The listing builds one solid part. Answer for the finished solid, in the listing's coordinates (mm). Round coordinates to 2 decimals unless told otherwise and drop trailing zeros. Write each loop counter-clockwise with the first axis right and the second up, starting at its lowest first coordinate (ties: lowest second). Pieces come first, ordered by that corner, then holes. Notation, with made-up numbers: M 11.5,54.25 L 47.5,54.25 A17 cw 47.5,78.25 Z; hole C -21.75,-40 d3. An arc over 180 degrees is marked long. One line per item, written item: value. Start each with the question number.
(1) Consider probe 1 along Z at (x, y) = (138, 0.7); probe 2 along Z at (x, y) = (254, 1.85); probe 3 along Z at (x, y) = (268.5, 2). Determine where each line is inside the solid, lowest interval first.
(2) Given P1, Ø3, axis at x = 253.5, z = -110, coming from the +Y side; P2, Ø4.5, axis at x = 253.5, z = -45, coming from the +Y side; P3, Ø1.5, axis at y = 1.5, z = -4.5, coming from the +X side; P4, Ø1.5, axis at y = 2, z = -98, coming from the -X side, each flat-ended and moving along its own axis, determine where each tip first touches the part or whether it passes through.
(3) Section A-A (z = -74.5) is taken. Determine the outline of the cut face in (x, y), plus the area to 3 significant figures.
(4) Section D-D (x = 67) is taken. Determine the outline of the cut face in (y, z).
(5) Section B-B (x = 290) is taken. Determine the outline of the cut face in (y, z).
(6) Section C-C (y = 2.15) is taken. State how many separate pieces and enclosed holes the cut face has, plus the area to 3 significant figures.
```python
from build123d import *

# Parameters (mm, degrees)
ESQUISSE1_R      = 2.5
EXTRUSION1_DEPTH = 3
CONG_1_R         = 15
EXTRUSION2_REACH = 5
ESQUISSE2_W      = 300
ESQUISSE2_H      = 3
ESQUISSE2_W_2    = 3
ESQUISSE2_H_2    = 93
ESQUISSE3_R      = 2
EXTRUSION3_DEPTH = 3


with BuildPart() as part:
    # Esquisse1 → Extrusion1 (new body)
    with BuildSketch(Plane(origin=(0, 0, 0), x_dir=(1, 0, 0), z_dir=(0, 1, 0))):
        Polygon((0, 0), (24, 0), (24, 14), (306, 14), (306, 0), (330, 0), (330, 123), (0, 123), align=None)
        with Locations((10, 113)):
            Circle(ESQUISSE1_R, mode=Mode.SUBTRACT)
        with Locations((320, 113)):
            Circle(ESQUISSE1_R, mode=Mode.SUBTRACT)
        with Locations((10, 12)):
            Circle(ESQUISSE1_R, mode=Mode.SUBTRACT)
        with Locations((320, 12)):
            Circle(ESQUISSE1_R, mode=Mode.SUBTRACT)
        with BuildLine():
            Line((280, 93), (280, 54))
            ThreePointArc((280, 54), (290, 44), (300, 54))
            Line((300, 54), (300, 93))
            ThreePointArc((300, 93), (290, 103), (280, 93))
        make_face(mode=Mode.SUBTRACT)
        with BuildLine():
            Line((30, 93), (30, 54))
            ThreePointArc((30, 54), (40, 44), (50, 54))
            Line((50, 54), (50, 93))
            ThreePointArc((50, 93), (40, 103), (30, 93))
        make_face(mode=Mode.SUBTRACT)
    extrude(amount=EXTRUSION1_DEPTH)

    # Congé1
    cong_1_edges = [part.edges().sort_by_distance(p)[0] for p in [
        (0, 1.5, -123),
        (330, 1.5, -123),
        (330, 1.5, 0),
        (0, 1.5, 0),
    ]]
    fillet(cong_1_edges, radius=CONG_1_R)

    # Esquisse2 → Extrusion2 (cut, up to next)
    with BuildSketch(Plane(origin=(0, 3, 0), x_dir=(1, 0, 0), z_dir=(0, 1, 0)), mode=Mode.PRIVATE) as extrusion2_sk1:
        with Locations((165, 121.5)):
            Rectangle(ESQUISSE2_W, ESQUISSE2_H)
    extrusion2_tool1 = extrude(extrusion2_sk1.sketch, amount=-EXTRUSION2_REACH, mode=Mode.PRIVATE) & part.part
    add(extrusion2_tool1.solids().sort_by_distance((165, 3, -121.5))[0], mode=Mode.SUBTRACT)
    # Esquisse2 → Extrusion2 (cut, up to next)
    with BuildSketch(Plane(origin=(0, 3, 0), x_dir=(1, 0, 0), z_dir=(0, 1, 0)), mode=Mode.PRIVATE) as extrusion2_sk2:
        with Locations((1.5, 61.5)):
            Rectangle(ESQUISSE2_W_2, ESQUISSE2_H_2)
    extrusion2_tool2 = extrude(extrusion2_sk2.sketch, amount=-EXTRUSION2_REACH, mode=Mode.PRIVATE) & part.part
    add(extrusion2_tool2.solids().sort_by_distance((1.5, 3, -61.5))[0], mode=Mode.SUBTRACT)
    # Esquisse2 → Extrusion2 (cut, up to next)
    with BuildSketch(Plane(origin=(0, 3, 0), x_dir=(1, 0, 0), z_dir=(0, 1, 0)), mode=Mode.PRIVATE) as extrusion2_sk3:
        with Locations((328.5, 61.5)):
            Rectangle(ESQUISSE2_W_2, ESQUISSE2_H_2)
    extrusion2_tool3 = extrude(extrusion2_sk3.sketch, amount=-EXTRUSION2_REACH, mode=Mode.PRIVATE) & part.part
    add(extrusion2_tool3.solids().sort_by_distance((328.5, 3, -61.5))[0], mode=Mode.SUBTRACT)

    # Esquisse3 → Extrusion3 (cut)
    with BuildSketch(Plane(origin=(0, 3, 0), x_dir=(1, 0, 0), z_dir=(0, 1, 0))):
        with Locations((76.5, 110)):
            Circle(ESQUISSE3_R)
        with Locations((253.5, 110)):
            Circle(ESQUISSE3_R)
        with Locations((76.5, 24)):
            Circle(ESQUISSE3_R)
        with Locations((253.5, 24)):
            Circle(ESQUISSE3_R)
        with Locations((61.5, 110)):
            Circle(ESQUISSE3_R)
        with Locations((106.5, 110)):
            Circle(ESQUISSE3_R)
        with Locations((61.5, 87)):
            Circle(ESQUISSE3_R)
        with Locations((106.5, 87)):
            Circle(ESQUISSE3_R)
        with Locations((61.5, 47)):
            Circle(ESQUISSE3_R)
        with Locations((106.5, 47)):
            Circle(ESQUISSE3_R)
        with Locations((106.5, 24)):
            Circle(ESQUISSE3_R)
        with Locations((61.5, 24)):
            Circle(ESQUISSE3_R)
        with Locations((223.5, 87)):
            Circle(ESQUISSE3_R)
        with Locations((223.5, 110)):
            Circle(ESQUISSE3_R)
        with Locations((268.5, 110)):
            Circle(ESQUISSE3_R)
        with Locations((268.5, 87)):
            Circle(ESQUISSE3_R)
        with Locations((268.5, 47)):
            Circle(ESQUISSE3_R)
        with Locations((268.5, 24)):
            Circle(ESQUISSE3_R)
        with Locations((223.5, 24)):
            Circle(ESQUISSE3_R)
        with Locations((223.5, 47)):
            Circle(ESQUISSE3_R)
        with Locations((191.5, 110)):
            Circle(ESQUISSE3_R)
        with Locations((191.5, 45)):
            Circle(ESQUISSE3_R)
        with Locations((138.5, 45)):
            Circle(ESQUISSE3_R)
        with Locations((138.5, 110)):
            Circle(ESQUISSE3_R)
        with Locations((76.5, 45)):
            Circle(ESQUISSE3_R)
        with Locations((253.5, 45)):
            Circle(ESQUISSE3_R)
    extrude(amount=-EXTRUSION3_DEPTH, mode=Mode.SUBTRACT)


solid = part.part
```
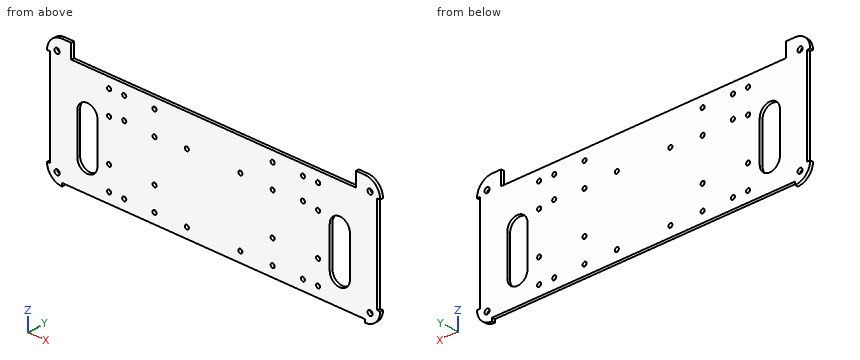
Recorded:
1. probe 1: z = -120 to -111.94, -108.06 to -46.94, -43.06 to -14
1. probe 2: z = -120 to -111.94, -108.06 to -46.94, -43.06 to -25.94, -22.06 to -14
1. probe 3: z = -120 to -112, -108 to -89, -85 to -49, -45 to -26, -22 to -14
2. P1: passes through
2. P2: stops at y = 3
2. P3: stops at x = 326.4
2. P4: stops at x = 3
3. outline: M 3,0 L 30,0 L 30,3 L 3,3 Z; M 50,0 L 280,0 L 280,3 L 50,3 Z; M 300,0 L 327,0 L 327,3 L 300,3 Z
3. area: 852 mm2
4. outline: M 0,-120 L 3,-120 L 3,-14 L 0,-14 Z
5. outline: M 0,-120 L 3,-120 L 3,-103 L 0,-103 Z; M 0,-44 L 3,-44 L 3,-14 L 0,-14 Z
6. separate pieces: 1
6. enclosed holes: 32
6. area: 32,400 mm2
